from build123d import *

# Parameters (mm, degrees)
F1_DEPTH = 10
F2_R     = 2
F4_D     = 4
F4_DEPTH = 15
F4_TIP   = 1.2017212381


with BuildPart() as f1:
    # F0 (on Top) → F1 (new body)
    with BuildSketch(Plane.XY):
        with BuildLine():
            Line((0, -22), (0, 0))
            Line((0, 0), (0, 22))
            Line((0, 22), (-4, 22))
            Line((-4, 22), (-4, 10))
            ThreePointArc((-4, 10), (-5.7573593129, 5.7573593129), (-10, 4))
            Line((-10, 4), (-22, 4))
            Line((-22, 4), (-22, 0))
            Line((-22, 0), (-22, -4))
            Line((-22, -4), (-10, -4))
            ThreePointArc((-10, -4), (-5.7573593129, -5.7573593129), (-4, -10))
            Line((-4, -10), (-4, -22))
            Line((-4, -22), (0, -22))
        make_face()
    extrude(amount=F1_DEPTH)

    # F2
    f2_edges = [f1.edges().sort_by_distance(p)[0] for p in [
        (-5.757359, -5.757359, 10),
        (-4, 16, 10),
        (-5.757359, -5.757359, 0),
        (-5.757359, 5.757359, 0),
    ]]
    fillet(f2_edges, radius=F2_R)

    # F4
    with Locations(Plane(origin=(-22, 0, 0), x_dir=(0, -1, 0), z_dir=(-1, 0, 0))):
        with Locations((0, 5)):
            Hole(F4_D / 2, depth=F4_DEPTH)
            with Locations((0, 0, -(F4_DEPTH + F4_TIP / 2))):  # 118° drill point
                Cone(0, F4_D / 2, F4_TIP, mode=Mode.SUBTRACT)


solid = f1.part
The model under review builds one solid part; all positions refer to its coordinate system, in mm. A direction names the side the tool comes from. Round coordinates to 2 decimals unless told otherwise and drop trailing zeros. Order: outer loops, then holes, each group sorted by start corner. A loop starts at its lowest first (then second) coordinate and runs counter-clockwise, first axis right, second up. Notation, with made-up numbers: (-39.75, 81.25) -> (-25.75, 81.25) arc R25 cw to (-25.75, 93.25) -> close; hole circle Ø11 at (-1.5, -1.5). An arc over 180 degrees is marked (long way). Return JSON: item names as keys, results as strings.
1. Take a section at B-B (z = 1). Write out the cut boundary in (x, y), then the cut area to 3 significant figures.
Answer block:
{"outline": "(-22, -3.73) -> (-10, -3.73) arc R6.27 cw to (-3.73, -10) -> (-3.73, -22) -> (0, -22) -> (0, 22) -> (-3.73, 22) -> (-3.73, 10) arc R6.27 cw to (-10, 3.73) -> (-22, 3.73) -> close", "area": "317 mm²"}
2. Take a section at A-A (x = -17.25). Write out the cut boundary in (y, z), then the cut area to 3 significant figures.
Answer block:
{"outline": "(-4, 2) arc R2 ccw to (-2, 0) -> (2, 0) arc R2 ccw to (4, 2) -> (4, 8) arc R2 ccw to (2, 10) -> (-2, 10) arc R2 ccw to (-4, 8) -> close; hole circle Ø4 at (0, 5)", "area": "64.0 mm²"}
3. Take a section at C-C (y = 17). Write out the cut boundary in (x, z).
Answer block:
{"outline": "(-4, 2) arc R2 ccw to (-2, 0) -> (0, 0) -> (0, 10) -> (-2, 10) arc R2 ccw to (-4, 8) -> close"}
4. The part is to be moulded in two halves that separate along Y. For faces 1 (the face through (-16, 4, 5)), 2 (the face through (-6.007, -0.187, 5.293)), 3 (the face through (-14, 0, 7)), 4 (the face through (-6, 0, 0)), say which applies: +Y half, -Y half, draft (parallel to the pull), parting line (faces both ways), or undercut.
Answer block:
{"face 1": "+Y half", "face 2": "undercut", "face 3": "undercut", "face 4": "draft"}
5. For faces 5 (the face through (-4, 16, 5)), 6 (the face through (-3.43, 15.92, 9.4)), 7 (the face through (-16.08, 3.43, 0.6)), 8 (the face through (-15.92, -3.43, 9.4)), 9 (the face through (-4, -16, 5)), list the 3-axis set-ups (+Z, -Z, +X, -X, +Y, -Y) from which the entire face can be reached by the end or side of a thin tool; tool diameter is ignored.
Answer block:
{"face 5": "+Z, -Z, -X, +Y", "face 6": "+Z, -X, +Y", "face 7": "-Z, -X, +Y", "face 8": "+Z, -X, -Y", "face 9": "+Z, -Z, -X, -Y"}
6. Insertion check: P1, Ø4, axis at x = -7.5, z = 5, coming from the -Y side; P2, Ø1.8, axis at y = -17.5, z = 4, coming from the -X side; P3, Ø2.5, axis at y = 0, z = 5, coming from the -X side. Each pin has a flat end and moves straight along its axis. Give the tip position at first contact, or say it passes through.
Answer block:
{"P1": "stops at y = -6.03", "P2": "stops at x = -4", "P3": "stops at x = -6.55"}
7. For L1, parallel to Y at x = -9.75, z = 5; L2, parallel to Z at x = -11.25, y = 0; L3, parallel to X at y = 20.5, z = 3.25, list the stretches that pass through material, from the lowest coordinate up. Write a range as [from, to].
Answer block:
{"L1": "y = [-4.01, -2], [2, 4.01]", "L2": "z = [0, 3], [7, 10]", "L3": "x = [-4, 0]"}
